Check sheet for the drawn part. Datum: minimum x, y, z corner. Units: mm. A direction names the side the tool comes from. Give positions to 0.01 mm unless a question says otherwise; leave off trailing zeros. Loops run counter-clockwise (first coordinate to the right, second up) from the corner with the lowest first, then second, coordinate; pieces in that order, holes last. Notation, with made-up numbers: M -18,-14.75 L 16,-14.75 A19 cw 16,-2.75 Z; hole C 87,21 d10. An arc over 180 degrees is marked long. Write each question's results on one line, items separated by ' | '. Start each with the question number.
1. Material ranges on line 1 along Z through (x, y) = (8, 14.25); line 2 along Z through (x, y) = (16, 20.75); line 3 along Y through (x, z) = (13, 12.75), recorded low to high.
2. Sectioned sample at B-B on y = 12.7. Record the cut outline in (x, z).
3. Sectioned sample at C-C on z = 12.75. Record the cut outline in (x, y).
4. Sectioned sample at D-D on y = 17. Record the cut outline in (x, z).
5. Tool access check on the marked faces 1, 2 and 3. Record the directions out of +Z, -Z, +X, -X, +Y, -Y that give a thin tool (end or side, any length) a straight path to the whole face; none if there is none.
6. Go/stop test with flat-tipped pins: pin 1 (3.5 mm diameter, centred on x = 13, z = 23, fed in from +Y); pin 2 (8 mm diameter, centred on x = 9.5, z = 13, fed in from +Y); pin 3 (3 mm diameter, centred on x = 6.5, z = 13.5, fed in from -Y). Record where each tip stops, or that it passes through.
7. Sectioned sample at A-A on x = 12.7. Record the cut outline in (y, z).
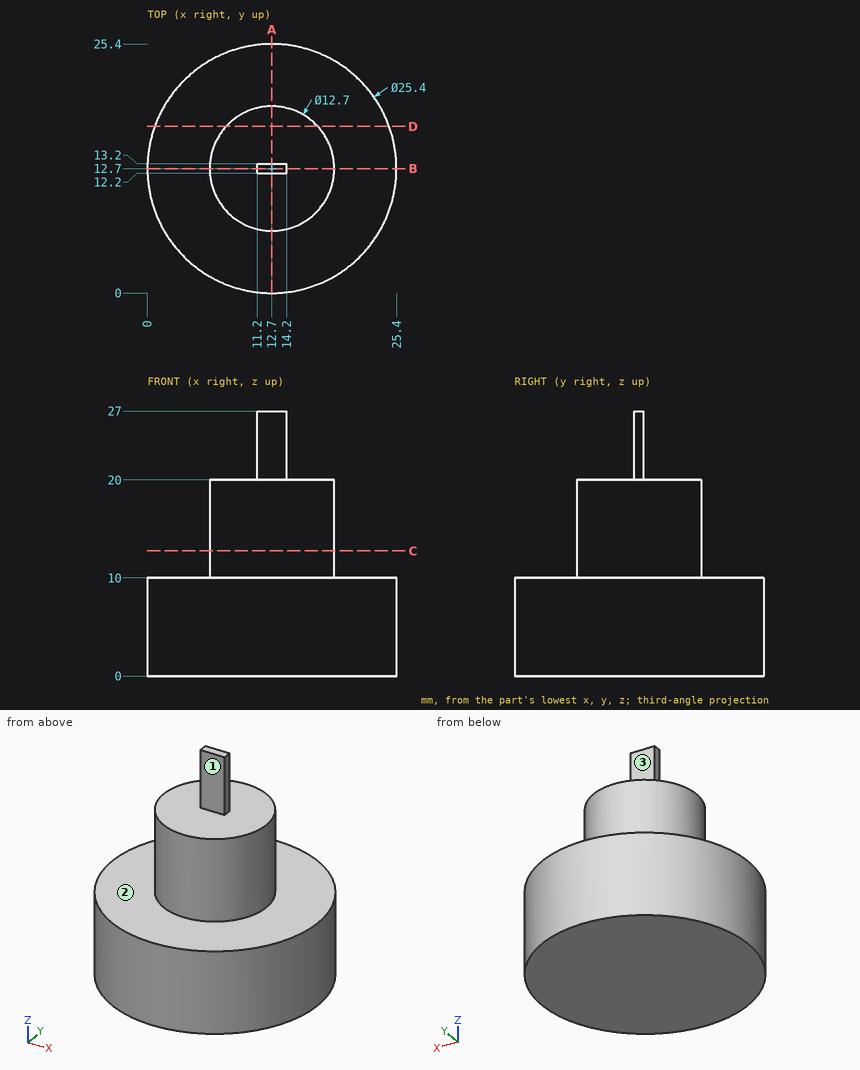
Output values:
1) line 1: 0 to 20 | line 2: 0 to 10 | line 3: 6.36 to 19.04
2) outline: M 0,0 L 25.4,0 L 25.4,10 L 19.05,10 L 19.05,20 L 14.2,20 L 14.2,27 L 11.2,27 L 11.2,20 L 6.35,20 L 6.35,10 L 0,10 Z
3) outline: C 12.7,12.7 d12.7
4) outline: M 0.75,0 L 24.65,0 L 24.65,10 L 17.37,10 L 17.37,20 L 8.03,20 L 8.03,10 L 0.75,10 Z
5) face 1: +Z, +X, -X, -Y | face 2: +Z | face 3: +Z, +X, -X, +Y
6) pin 1: y = 13.2 | pin 2: y = 25.39 | pin 3: y = 8.43
7) outline: M 0,0 L 25.4,0 L 25.4,10 L 19.05,10 L 19.05,20 L 13.2,20 L 13.2,27 L 12.2,27 L 12.2,20 L 6.35,20 L 6.35,10 L 0,10 Z
